Build history of the part. All positions in model axes, mm. Give positions to 0.01 mm unless a question says otherwise; leave off trailing zeros. Write each loop counter-clockwise with the first axis right and the second up, starting at its lowest first coordinate (ties: lowest second). Pieces come first, ordered by that corner, then holes.
from build123d import *

# Parameters (mm, degrees)
BASE_FLANGE1_DEPTH = 450
SKETCH3_R          = 2.25425
CUT_EXTRUDE1_DEPTH = 1.4


# Sheet-metal steps are written as plain solids
with BuildPart() as part:
    # Sketch2 → Base-Flange1 (new body)
    with BuildSketch(Plane(origin=(0, 0, 0), x_dir=(0, 0, -1), z_dir=(1, 0, 0))):
        with BuildLine():
            Line((1.875, 7.1), (1.875, 1.85))
            ThreePointArc((1.875, 1.85), (1.948223305, 1.673223305), (2.125, 1.6))
            Line((2.125, 1.6), (22.125, 1.6))
            ThreePointArc((22.125, 1.6), (22.301776695, 1.673223305), (22.375, 1.85))
            Line((22.375, 1.85), (22.375, 7.1))
            Line((22.375, 7.1), (23.775, 7.1))
            Line((23.775, 7.1), (23.775, 1.85))
            ThreePointArc((23.775, 1.85), (23.291726189, 0.683273811), (22.125, 0.2))
            Line((22.125, 0.2), (2.125, 0.2))
            ThreePointArc((2.125, 0.2), (0.958273811, 0.683273811), (0.475, 1.85))
            Line((0.475, 1.85), (0.475, 7.1))
            Line((0.475, 7.1), (1.875, 7.1))
        make_face()
    extrude(amount=BASE_FLANGE1_DEPTH)

    # Sketch3 → Cut-Extrude1 (cut)
    with BuildSketch(Plane.XZ.offset(-0.2)):
        with Locations(Location((25.4, -12.125, 0), (0, 0, 270))):
            Circle(SKETCH3_R)
        with Locations(Location((50.8, -12.125, 0), (0, 0, 270))):
            Circle(SKETCH3_R)
        with Locations(Location((215.9, -12.125, 0), (0, 0, 270))):
            Circle(SKETCH3_R)
        with Locations(Location((190.5, -12.125, 0), (0, 0, 270))):
            Circle(SKETCH3_R)
    extrude(amount=-CUT_EXTRUDE1_DEPTH, mode=Mode.SUBTRACT)


solid = part.part
1. Mould opens along Z. For faces 1 (the face through (222, 1.6, -12)), 2 (the face through (450, 1, -12)) say: pulls with the +Z half, pulls with the -Z half, needs draft (parallel to the pull), parting line crosses it, or undercut.
2. Saw through at B-B on x = 77. Give the cut face in (y, z) (3 decimals), plus the area to 3 significant figures.
3. Drill centre lines: line 1 along Z through (x, y) = (319, 5.5) (3 decimals); line 2 along X through (y, z) = (0.75, -13.5); line 3 along Y through (x, z) = (305.5, -3). Where is each one in solid material? Low to high.
4. Drop flat-ended pins along their axis: pin 1 (10 mm diameter, centred on x = 212, z = -13.5, fed in from +Y); pin 2 (1.5 mm diameter, centred on y = 4, z = -13.5, fed in from -X); pin 3 (4 mm diameter, centred on x = 212.5, y = 1, fed in from +Z) (3 decimals). Give the stop position or say it passes through.
5. Saw through at A-A on y = 4.5. Give the cut face in (x, z) (3 decimals), plus the area to 3 significant figures.
Outcome:
1. face 1: undercut
1. face 2: needs draft
2. outline: (0.2, -22.125) arc R1.65 ccw to (1.85, -23.775) - (7.1, -23.775) - (7.1, -22.375) - (1.85, -22.375) arc R0.25 cw to (1.6, -22.125) - (1.6, -2.125) arc R0.25 cw to (1.85, -1.875) - (7.1, -1.875) - (7.1, -0.475) - (1.85, -0.475) arc R1.65 ccw to (0.2, -2.125) - close
2. area: 46.9 mm2
3. line 1: z = -23.775 to -22.375, -1.875 to -0.475
3. line 2: x = 0 to 23.61, 27.19 to 49.01, 52.59 to 188.71, 192.29 to 214.11, 217.69 to 450
3. line 3: y = 0.2 to 1.6
4. pin 1: stops at y = 1.6
4. pin 2: passes through
4. pin 3: stops at z = -0.475
5. outline: (0, -23.775) - (450, -23.775) - (450, -22.375) - (0, -22.375) - close; (0, -1.875) - (450, -1.875) - (450, -0.475) - (0, -0.475) - close
5. area: 1,260 mm2
